Can you work these out from the model? Positions are in its coordinate system, mm. Face numbers are marked on the shaded views. Give positions to 0.01 mm unless a question says otherwise; leave off trailing zeros. Order: outer loops, then holes, each group sorted by start corner. A loop starts at its lowest first (then second) coordinate and runs counter-clockwise, first axis right, second up. Notation, with made-up numbers: (-7.75, -32.5) - (14.25, -32.5) arc R13 ccw to (14.25, -25.5) - close; hole circle Ø3 at (9.5, 21). An arc over 180 degrees is marked (long way). One line per question, with ' | ' between items.
```python
from build123d import *

# Parameters (mm, degrees)
SKETCH1_R           = 22.4
SKETCH1_R_2         = 10
BOSS_EXTRUDE1_DEPTH = 12
CUT_EXTRUDE1_START  = -0.5
SKETCH2_R           = 22.4
SKETCH2_R_2         = 20.9
CUT_EXTRUDE1_DEPTH  = 0.5
FILLET1_R           = 0.1
FILLET2_R           = 0.1
SKETCH3_R           = 1.5
CUT_EXTRUDE2_DEPTH  = 12


with BuildPart() as part:
    # Sketch1 → Boss-Extrude1 (new body)
    with BuildSketch(Plane(origin=(0, 0, 0), x_dir=(1, 0, 0), z_dir=(0, 1, 0))):
        with Locations(Location((0, 0, 0), (0, 0, 270))):
            Circle(SKETCH1_R)
        with Locations(Location((0, 0, 0), (0, 0, 270))):
            Circle(SKETCH1_R_2, mode=Mode.SUBTRACT)
    extrude(amount=BOSS_EXTRUDE1_DEPTH)

    # Sketch2 → Cut-Extrude1 (cut)
    with BuildSketch(Plane(origin=(0, 12, 0), x_dir=(1, 0, 0), z_dir=(0, 1, 0)).offset(CUT_EXTRUDE1_START)):
        with Locations(Location((0, 0, 0), (0, 0, 270))):
            Circle(SKETCH2_R)
        with Locations(Location((0, 0, 0), (0, 0, 270))):
            Circle(SKETCH2_R_2, mode=Mode.SUBTRACT)
    cut_extrude1 = extrude(amount=CUT_EXTRUDE1_DEPTH, mode=Mode.SUBTRACT)

    # Fillet1
    fillet1_edges = [part.edges().sort_by_distance(p)[0] for p in [
        (0, 12, -20.9),
    ]]
    fillet(fillet1_edges, radius=FILLET1_R)

    # Mirror3: Cut-Extrude1 across plane
    add(cut_extrude1.mirror(Plane.ZX.offset(6)), mode=Mode.SUBTRACT)

    # Fillet2
    fillet2_edges = [part.edges().sort_by_distance(p)[0] for p in [
        (0, 0, -20.9),
    ]]
    fillet(fillet2_edges, radius=FILLET2_R)

    # Sketch3 → Cut-Extrude2 (cut)
    with BuildSketch(Plane(origin=(0, 12, 0), x_dir=(1, 0, 0), z_dir=(0, 1, 0))):
        with Locations(Location((0, 14, 0), (0, 0, 270))):
            Circle(SKETCH3_R)
        with Locations(Location((12.124355653, 7, 0), (0, 0, 270))):
            Circle(SKETCH3_R)
        with Locations(Location((12.124355653, -7, 0), (0, 0, 270))):
            Circle(SKETCH3_R)
        with Locations(Location((0, -14, 0), (0, 0, 270))):
            Circle(SKETCH3_R)
        with Locations(Location((-12.124355653, -7, 0), (0, 0, 270))):
            Circle(SKETCH3_R)
        with Locations(Location((-12.124355653, 7, 0), (0, 0, 270))):
            Circle(SKETCH3_R)
    extrude(amount=-CUT_EXTRUDE2_DEPTH, mode=Mode.SUBTRACT)


solid = part.part
```
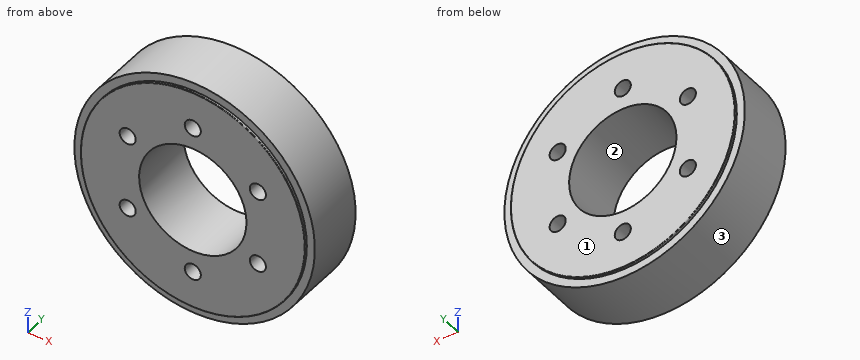
(1) Imagine slicing it at B-B (x = 0). List the corners of the cut face in (y, z) for me, and give its area (3 significant figures).
Answer below:
outline: (0, -20.8) arc R0.1 ccw to (0.1, -20.9) - (0.5, -20.9) - (0.5, -22.4) - (11.5, -22.4) - (11.5, -20.9) - (11.9, -20.9) arc R0.1 ccw to (12, -20.8) - (12, -15.5) - (0, -15.5) - close; (0, -12.5) - (12, -12.5) - (12, -10) - (0, -10) - close; (0, 10) - (12, 10) - (12, 12.5) - (0, 12.5) - close; (0, 15.5) - (12, 15.5) - (12, 20.8) arc R0.1 ccw to (11.9, 20.9) - (11.5, 20.9) - (11.5, 22.4) - (0.5, 22.4) - (0.5, 20.9) - (0.1, 20.9) arc R0.1 ccw to (0, 20.8) - close | area: 223 mm^2
(2) Will these pins go through, and if not, where does the flat tip stop? pin 1 (5 mm diameter, centred on x = 12.12, z = 7, fed in from -Y); pin 2 (1 mm diameter, centred on y = 5, z = -14, fed in from -X); pin 3 (2.5 mm diameter, centred on x = -12.12, z = 7, fed in from -Y); pin 4 (5 mm diameter, centred on y = 9, z = -11, fed in from +X).
Answer below:
pin 1: y = 0 | pin 2: x = -17.87 | pin 3: through | pin 4: x = 20.72
(3) Imagine slicing it at C-C (y = 1.5). List the corners of the cut face in (x, z) for me.
Answer below:
outline: circle Ø44.8 at (0, 0); hole circle Ø3 at (-12.12, -7); hole circle Ø3 at (-12.12, 7); hole circle Ø20 at (0, 0); hole circle Ø3 at (0, -14); hole circle Ø3 at (0, 14); hole circle Ø3 at (12.12, -7); hole circle Ø3 at (12.12, 7)
(4) If we mould it in two halves opening along Z, with no side actions, what happens to the marked faces 1, 2 and 3? For each: released by +Z, released by -Z, zero draft, split by the parting line, or undercut.
Answer below:
face 1: zero draft | face 2: undercut | face 3: split by the parting line
(5) If I drill on line 1 (Z direction, x = -11.5, y = 11.75); line 2 (Z direction, x = 7, y = 7.75); line 3 (Z direction, x = -9, y = 4.25), over which ranges is the centre line in solid material (lowest first)?
Answer below:
line 1: -17.45 to -8.36, -5.64 to 5.64, 8.36 to 17.45 | line 2: -21.28 to -7.14, 7.14 to 21.28 | line 3: -20.51 to -4.36, 4.36 to 20.51
(6) Imagine slicing it at D-D (z = 7). Count the separate pieces of the cut face and the enclosed holes in it, and give its area (3 significant figures).
Answer below:
separate pieces: 4 | enclosed holes: 0 | area: 264 mm^2
(7) Imagine slicing it at A-A (z = 0). List the corners of the cut face in (x, y) for me.
Answer below:
outline: (-22.4, 0.5) - (-20.9, 0.5) - (-20.9, 0.1) arc R0.1 ccw to (-20.8, 0) - (-10, 0) - (-10, 12) - (-20.8, 12) arc R0.1 ccw to (-20.9, 11.9) - (-20.9, 11.5) - (-22.4, 11.5) - close; (10, 0) - (20.8, 0) arc R0.1 ccw to (20.9, 0.1) - (20.9, 0.5) - (22.4, 0.5) - (22.4, 11.5) - (20.9, 11.5) - (20.9, 11.9) arc R0.1 ccw to (20.8, 12) - (10, 12) - close
